Can you work these out from the drawing? Everything is in mm from the part's minimum corner. A direction names the side the tool comes from. Coordinates: 2 decimals unless noted, no trailing zeros. Loops run counter-clockwise (first coordinate to the right, second up) from the corner with the lowest first, then second, coordinate; pieces in that order, holes last.
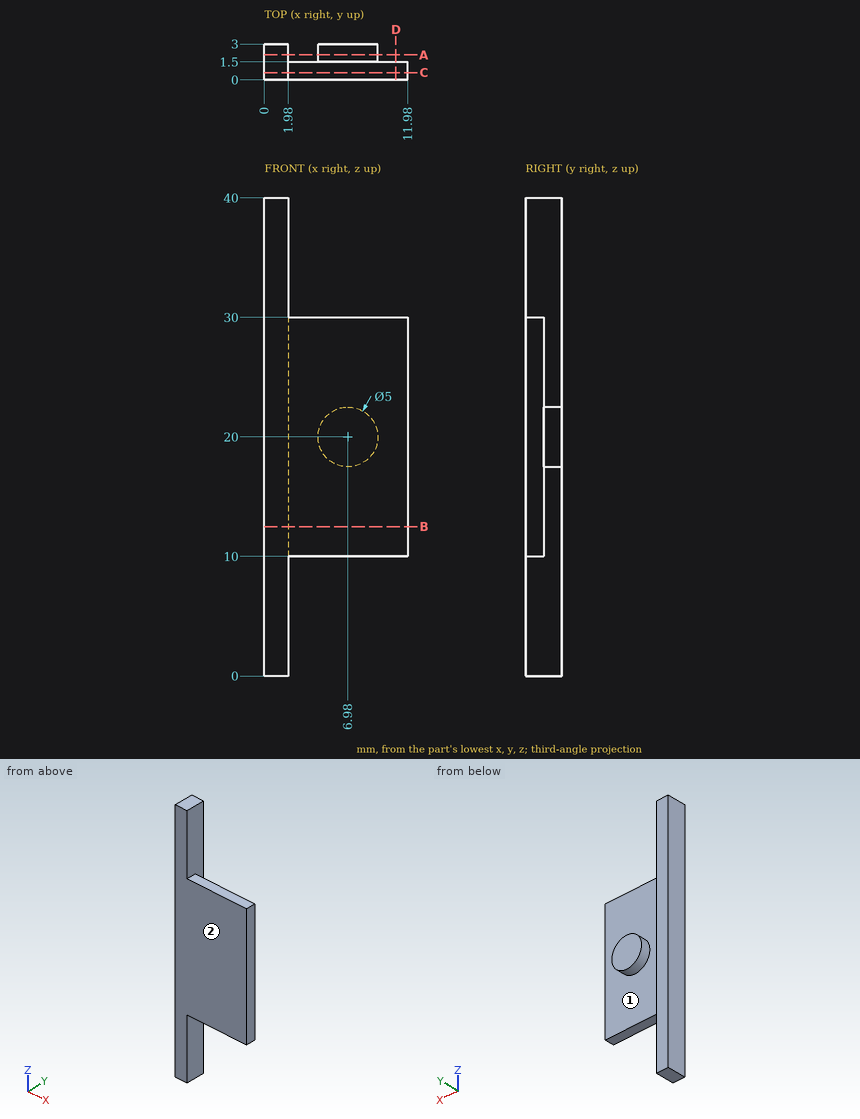
Item 1: On a 3-axis mill with a long thin cutter (end or side, diameter ignored), from which of +Z, -Z, +X, -X, +Y, -Y can I reach the whole of each face in a straight line? I mean the marked faces 1 and 2. Say none if no direction works.
Results are:
face 1: +Y
face 2: +Z, -Z, +X, -X, -Y
Item 2: Suppose I cut it at D-D, the plane x = 11. Please give me the cut outline in (y, z), plus the area to 3 significant figures.
Results are:
outline: (0, 10) - (1.5, 10) - (1.5, 30) - (0, 30) - close
area: 30.0 mm2
Item 3: I'm going to push flat-ended pins straight in: P1, Ø0.8, axis at x = 6.5, y = 0.5, coming from the +Z side; P2, Ø1.5, axis at x = 8.5, z = 23.5, coming from the +Y side; P3, Ø6, axis at x = 9.5, z = 35, coming from the -Y side. Where does each tip first touch, or does it pass through?
Results are:
P1: stops at z = 30
P2: stops at y = 1.5
P3: passes through
Item 4: I need wall thicknesses on line 1 along Y through (x, z) = (8.75, 25); line 2 along X through (y, z) = (1.25, 38); line 3 along Z through (x, y) = (11.25, 0.2). Which ranges of each line are inside material? Lowest first, please.
Results are:
line 1: y = 0 to 1.5
line 2: x = 0 to 1.98
line 3: z = 10 to 30
Item 5: Suppose I cut it at C-C, the plane y = 0.6. Please give me the cut outline in (x, z), plus the area to 3 significant figures.
Results are:
outline: (0, 0) - (1.98, 0) - (1.98, 10) - (11.98, 10) - (11.98, 30) - (1.98, 30) - (1.98, 40) - (0, 40) - close
area: 279 mm2
Item 6: Suppose I cut it at A-A, the plane y = 2.1. Please give me the cut outline in (x, z).
Results are:
outline: (0, 0) - (1.98, 0) - (1.98, 40) - (0, 40) - close; circle Ø5 at (6.98, 20)
Item 7: Suppose I cut it at B-B, the plane z = 12.5. Please give me the cut outline in (x, y).
Results are:
outline: (0, 0) - (11.98, 0) - (11.98, 1.5) - (1.98, 1.5) - (1.98, 3) - (0, 3) - close
